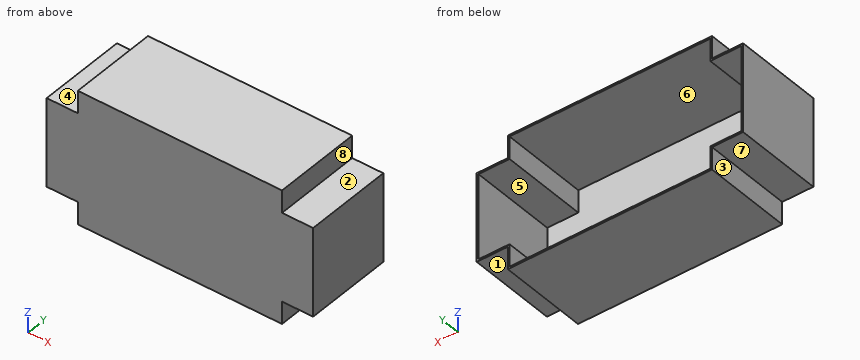
Autodesk Inventor part; units mm, degrees
ref_plane "Work Plane3" through (133.62, 1, -38.1) normal (0, 0, -1) x (-1, 0, 0)
ref_plane "YZ Plane" through (0, 0, 0) normal (1, 0, 0) x (0, 1, 0)
ref_plane "XZ Plane" through (0, 0, 0) normal (0, 1, 0) x (-1, 0, 0)
sketch "Sketch1" plane through (0, 0, 0) normal (0, 0, 1) x (1, 0, 0)
  line L0 (0, 0) -> (152.4, 0)
  line L1 (152.4, 0) -> (152.4, 50.8)
  line L2 (152.4, 50.8) -> (0, 50.8)
  line L3 (0, 50.8) -> (0, 0)
  line L4 (0, 50.8) -> (17.78, 50.8)
  line L5 (17.78, 0) -> (0, 0)
  line L6 (0, 0) -> (0, 50.8)
  line L7 (152.4, 0) -> (134.62, 0)
  line L8 (134.62, 50.8) -> (152.4, 50.8)
  line L9 (152.4, 50.8) -> (152.4, 0)
  dimension "d0" = 152.4
  dimension "d1" = 50.8
extrude "Extrusion1" add sketch "Sketch1" against normal blind 38.1
sketch "Sketch2" plane through (0, 0, 0) normal (0, 0, 1) x (1, 0, 0)
  line L0 (0, 50.8) -> (152.4, 50.8)
  line L1 (152.4, 0) -> (0, 0)
  line L2 (0, 50.8) -> (17.78, 50.8)
  line L3 (17.78, 50.8) -> (17.78, 0)
  line L4 (17.78, 0) -> (0, 0)
  line L5 (0, 0) -> (0, 50.8)
  line L6 (152.4, 0) -> (134.62, 0)
  line L7 (134.62, 0) -> (134.62, 50.8)
  line L8 (134.62, 50.8) -> (152.4, 50.8)
  line L9 (152.4, 50.8) -> (152.4, 0)
  point P0 (134.62, 0)
  dimension "d6" = 17.78
  dimension "d7" = 17.78
extrude "Extrusion2" cut sketch "Sketch2" against normal blind 12.8 contours L0 L3 L1 L5 | L0 L9 L1 L7
shell "Shell1" thickness 1 removed faces 2 at (56.7267, 50.8, -29.6667) at (101.6, 16.9333, -38.1)
ref_plane "Work Plane3" through (133.62, 1, -38.1) normal (0, 0, -1) x (-1, 0, 0)
mirror "Mirror2" about plane through (133.62, 1, -38.1) normal (0, 0, -1) of "Extrusion1", "Extrusion2"
shell "Shell6" thickness 1 removed faces 2 at (95.6733, 50.8, -46.5333) at (101.2667, 17.6, -38.1)
properties part number "Footprint"
Part model, mm, in its own coordinate system. Face numbers are marked on the shaded views. A direction names the side the tool comes from. Give positions to 0.01 mm unless a question says otherwise; leave off trailing zeros. Order: outer loops, then holes, each group sorted by start corner. A loop starts at its lowest first (then second) coordinate and runs counter-clockwise, first axis right, second up. Notation, with made-up numbers: (21.5, 70) - (79.5, 70) arc R27 cw to (79.5, 92) - close; hole circle Ø5 at (5.5, 70). An arc over 180 degrees is marked (long way). Use one line per item in the form item = value.
Item 1: Slice it at A-A on y = 11. Give the cut face in (x, z).
Solution:
outline = (0, -63.4) - (17.78, -63.4) - (17.78, -76.2) - (134.62, -76.2) - (134.62, -63.4) - (152.4, -63.4) - (152.4, -12.8) - (134.62, -12.8) - (134.62, 0) - (17.78, 0) - (17.78, -12.8) - (0, -12.8) - close; hole (1, -62.4) - (18.78, -62.4) - (18.78, -75.2) - (133.62, -75.2) - (133.62, -62.4) - (151.4, -62.4) - (151.4, -13.8) - (133.62, -13.8) - (133.62, -1) - (18.78, -1) - (18.78, -13.8) - (1, -13.8) - close
Item 2: Pin check, flat tips, straight feed: pin 1 Ø6.5 at (y, z) = (13, -9) entering from -X; pin 2 Ø14 at (x, y) = (147.5, 22) entering from -Z; pin 3 Ø6.5 at (y, z) = (20.5, -68.5) entering from +X. Stop position of each tip, or through.
Solution:
pin_1 = 17.78
pin_2 = -63.4
pin_3 = 134.62
Item 3: Probe probe 1 along Z at (x, y) = (106.5, 9); probe 2 along X at (y, z) = (12.5, -8.5); probe 3 along X at (y, z) = (12.5, -21). List the from-to ranges inside material, lowest first. Write a range as from..to.
Solution:
probe_1 = -76.2..-75.2, -1..0
probe_2 = 17.78..18.78, 133.62..134.62
probe_3 = 0..1, 151.4..152.4
Item 4: Which spindle directions (+Z, -Z, +X, -X, +Y, -Y) get a long thin tool onto all of the face, cutting with end or side? Do the marked faces 1, 2, 3, 4 and 5. Say none if no direction does.
Solution:
face_1 = -Z, +X, +Y, -Y
face_2 = +Z, +X, +Y, -Y
face_3 = -Z, -X, +Y, -Y
face_4 = +Z, -X, +Y, -Y
face_5 = +Y
Item 5: Slice it at C-C on z = -45. Give the cut face in (x, y), and give its area (3 significant figures).
Solution:
outline = (0, 0) - (152.4, 0) - (152.4, 50.8) - (151.4, 50.8) - (151.4, 1) - (1, 1) - (1, 50.8) - (0, 50.8) - close
area = 252 mm2
Item 6: Slice it at B-B on x = 25. Give the cut face in (y, z).
Solution:
outline = (0, -76.2) - (50.8, -76.2) - (50.8, -75.2) - (1, -75.2) - (1, -1) - (50.8, -1) - (50.8, 0) - (0, 0) - close
Item 7: Two-plate mould, pull along X, no slides. Class the marked faces 6, 7 and 8: released by +X, released by -X, zero draft, split by the parting line, or undercut.
Solution:
face_6 = undercut
face_7 = zero draft
face_8 = released by +X
